The listing builds one solid part. Answer for the finished solid, in the listing's coordinates (mm). A direction names the side the tool comes from. Round coordinates to 2 decimals unless told otherwise and drop trailing zeros. Loops run counter-clockwise (first coordinate to the right, second up) from the corner with the lowest first, then second, coordinate; pieces in that order, holes last. Notation, with made-up numbers: (-12, 4.5) - (26, 4.5) arc R36 cw to (26, 43.5) - close; hole circle Ø9 at (-30, 62). An arc over 180 degrees is marked (long way). One line per item, written item: value.
```python
from build123d import *

# Parameters (mm, degrees)
PAD001_DEPTH  = 50
PAD002_DEPTH  = 50
SKETCH005_W   = 14
SKETCH005_H   = 13
PAD004_DEPTH  = 20
SKETCH006_W   = 14
SKETCH006_H   = 13
PAD005_DEPTH  = 20
SKETCH007_W   = 14
SKETCH007_H   = 13
PAD006_DEPTH  = 20
SKETCH008_W   = 14
SKETCH008_H   = 13
PAD007_DEPTH  = 20
SKETCH003_W   = 32
SKETCH003_H   = 3
PAD003_DEPTH  = 50
SKETCH004_R   = 2.75
HOLE_DEPTH    = 3.001
SKETCH009_W   = 16
SKETCH009_H   = 29
PAD008_DEPTH  = 30
SKETCH010_R   = 6.6
HOLE001_DEPTH = 29.001
SKETCH011_W   = 16
SKETCH011_H   = 29
PAD009_DEPTH  = 24
SKETCH012_R   = 6.6
HOLE002_DEPTH = 29.001001
SKETCH_W      = 32
SKETCH_H      = 42
PAD_DEPTH     = 50
SKETCH014_R   = 6.6
HOLE004_DEPTH = 32.001
FILLET_R      = 8
FILLET001_R   = 8


with BuildPart() as body001:
    # Sketch001 (on Face1 of CopyPad) → Pad001 (new body)
    with BuildSketch(Plane.YZ.offset(50)):
        Polygon((19, 44), (32, 44), (32, 2), (27, 2), (19, 12.011942), align=None)
    extrude(amount=-PAD001_DEPTH)


with BuildPart() as body002:
    # Sketch002 (on Face1 of CopyPad001) → Pad002 (new body)
    with BuildSketch(Plane.YZ.offset(50)):
        Polygon((13, 44), (13, 12), (5, 2), (0, 2), (0, 44), align=None)
    extrude(amount=-PAD002_DEPTH)


with BuildPart() as body004:
    # Sketch005 (on Face1 of CopyHole) → Pad004 (new body)
    with BuildSketch(Plane.XY.offset(2)):
        with Locations((7, 6.5)):
            Rectangle(SKETCH005_W, SKETCH005_H)
    extrude(amount=PAD004_DEPTH)


with BuildPart() as body005:
    # Sketch006 (on Face1 of CopyHole001) → Pad005 (new body)
    with BuildSketch(Plane.XY.offset(2)):
        with Locations((7, 25.5)):
            Rectangle(SKETCH006_W, SKETCH006_H)
    extrude(amount=PAD005_DEPTH)


with BuildPart() as body006:
    # Sketch007 (on Face1 of CopyHole002) → Pad006 (new body)
    with BuildSketch(Plane.XY.offset(2)):
        with Locations((43, 6.5)):
            Rectangle(SKETCH007_W, SKETCH007_H)
    extrude(amount=PAD006_DEPTH)


with BuildPart() as body007:
    # Sketch008 (on Face1 of CopyHole003) → Pad007 (new body)
    with BuildSketch(Plane.XY.offset(2)):
        with Locations((43, 25.5)):
            Rectangle(SKETCH008_W, SKETCH008_H)
    extrude(amount=PAD007_DEPTH)


with BuildPart() as body003:
    # Sketch003 (on Face1 of CopyPad002) → Pad003 (new body)
    with BuildSketch(Plane(origin=(0, 0, 0), x_dir=(0, -1, 0), z_dir=(-1, 0, 0))):
        with Locations((-16, 0.5)):
            Rectangle(SKETCH003_W, SKETCH003_H)
    extrude(amount=-PAD003_DEPTH)

    # Sketch004 (on Face1 of Pad003) → Hole (cut, through all)
    with BuildSketch(Plane.XY.offset(2)):
        with Locations((5, 27)):
            Circle(SKETCH004_R)
        with Locations((5, 5)):
            Circle(SKETCH004_R)
        with Locations((45, 5)):
            Circle(SKETCH004_R)
        with Locations((45, 27.276354)):
            Circle(SKETCH004_R)
    extrude(amount=-HOLE_DEPTH, mode=Mode.SUBTRACT)


with BuildPart() as body008:
    # Sketch009 (on Face1 of CopyPad003) → Pad008 (new body)
    with BuildSketch(Plane(origin=(0, 0, 44), x_dir=(0, -1, 0), z_dir=(0, 0, 1))):
        with Locations((-16, 24.5)):
            Rectangle(SKETCH009_W, SKETCH009_H)
    extrude(amount=PAD008_DEPTH)

    # Sketch010 (on Face1 of Pad008) → Hole001 (cut, through all)
    with BuildSketch(Plane(origin=(10, 0, 0), x_dir=(0, 1, 0), z_dir=(-1, 0, 0))):
        with Locations((16, -59)):
            Circle(SKETCH010_R)
    extrude(amount=-HOLE001_DEPTH, mode=Mode.SUBTRACT)


with BuildPart() as body009:
    # Sketch011 (on Face1 of CopyHole001001) → Pad009 (new body)
    with BuildSketch(Plane.XY.offset(74)):
        with Locations((25, 16)):
            Rectangle(SKETCH011_W, SKETCH011_H)
    extrude(amount=PAD009_DEPTH)

    # Sketch012 (on Face1 of Pad009) → Hole002 (cut, through all)
    with BuildSketch(Plane(origin=(-1e-06, 30.5, 30.000001), x_dir=(-1, 0, 0), z_dir=(0, 1, 0))):
        with Locations((-25, 59)):
            Circle(SKETCH012_R)
    extrude(amount=-HOLE002_DEPTH, mode=Mode.SUBTRACT)


with BuildPart() as body:
    # Sketch → Pad (new body)
    with BuildSketch(Plane.YZ):
        with Locations((16, 23)):
            Rectangle(SKETCH_W, SKETCH_H)
    extrude(amount=PAD_DEPTH)

    # Sketch014 (on Face2 of Pad) → Hole004 (cut, through all)
    with BuildSketch(Plane.ZX.offset(32)):
        with Locations((28.082674, 37)):
            Circle(SKETCH014_R)
        with Locations((28, 13)):
            Circle(SKETCH014_R)
    extrude(amount=-HOLE004_DEPTH, mode=Mode.SUBTRACT)

    # Boolean: cut Body001
    add(body001.part, mode=Mode.SUBTRACT)

    # Boolean001: cut Body002
    add(body002.part, mode=Mode.SUBTRACT)

    # Boolean002: cut Body004
    add(body004.part, mode=Mode.SUBTRACT)

    # Boolean003: cut Body005
    add(body005.part, mode=Mode.SUBTRACT)

    # Boolean004: cut Body006
    add(body006.part, mode=Mode.SUBTRACT)

    # Boolean005: cut Body007
    add(body007.part, mode=Mode.SUBTRACT)

    # Boolean006: union Body003
    add(body003.part)

    # Boolean007: union Body008, Body009
    add(body008.part)
    add(body009.part)

    # Fillet
    fillet_edges = [body.edges().sort_by_distance(p)[0] for p in [
        (50, 16, 44),
    ]]
    fillet(fillet_edges, radius=FILLET_R)

    # Fillet001
    fillet001_edges = [body.edges().sort_by_distance(p)[0] for p in [
        (0, 16, 44),
    ]]
    fillet(fillet001_edges, radius=FILLET001_R)


solid = body.part
```
1) A cutting plane is placed at A-A on x = 13. Give the vertices of the cut face in (y, z), and give its area (3 significant figures).
Final values:
outline: (0, -1) - (32, -1) - (32, 2) - (19, 2) - (19, 21.4) - (13, 21.4) - (13, 2) - (0, 2) - close; (8, 44) - (13, 44) - (13, 34.6) - (19, 34.6) - (19, 44) - (24, 44) - (24, 74) - (8, 74) - close; hole circle Ø13.2 at (16, 59)
area: 612 mm2
2) Consider L1, parallel to Z at x = 37, y = 16.25; L2, parallel to Y at x = 45, z = 0.85; L3, parallel to Z at x = 25.5, y = 27. Determine where each line is inside the solid, lowest interval first.
Final values:
L1: -1 to 21.48, 34.68 to 52.4, 65.6 to 74
L2: 0 to 2.25, 7.75 to 24.53, 30.03 to 32
L3: -1 to 2, 74 to 82.42, 95.58 to 98
3) For faces 4 (the flat face through (24, 24, 59)), 5 (the flat face through (36, 22, 6)), 6 (the flat face through (25, 5, 74)), determine the directions among +Z, -Z, +X, -X, +Y, -Y from which every point of the face is accessible in a straight line to the end or side of a thin tool.
Final values:
face 4: +X, -X, +Y
face 5: +X, +Y
face 6: +X, -X, -Y
4) For a pull along Z with two mould halves and no side action, classify faces 1 (the flat face through (25, 16, 98)), 2 (the flat face through (25, 28, 2)), 3 (the flat face through (50, 16, 13)) as released by +Z, released by -Z, zero draft, split by the parting line, or undercut.
Final values:
face 1: released by +Z
face 2: undercut
face 3: zero draft
5) A cutting plane is placed at B-B on z = 59. Give the vertices of the cut face in (x, y).
Final values:
outline: (10, 8) - (39, 8) - (39, 9.4) - (10, 9.4) - close; (10, 22.6) - (39, 22.6) - (39, 24) - (10, 24) - close
6) A cutting plane is placed at C-C on y = 21. Give the vertices of the cut face in (x, z), and give its area (3 significant figures).
Final values:
outline: (0, -1) - (50, -1) - (50, 2) - (36, 2) - (36, 9.51) - (14, 9.51) - (14, 2) - (0, 2) - close; (10, 44) - (39, 44) - (39, 54.69) - (10, 54.69) - close; (10, 63.31) - (39, 63.31) - (39, 74) - (33, 74) - (33, 98) - (17, 98) - (17, 74) - (10, 74) - close; hole circle Ø13.2 at (25, 89)
area: 1,180 mm2
7) Each of these flat-tipped pins is pushed along its axis until it touches: pin 1 Ø5 at (x, z) = (24, 73) entering from +Y; pin 2 Ø10.5 at (x, z) = (37, 28.08) entering from -Y (1 decimal); pin 3 Ø6.5 at (y, z) = (8.5, 5.5) entering from -X; pin 4 Ø6 at (x, z) = (26.5, 40.5) entering from -Y. Where does it stop, or does it pass through?
Final values:
pin 1: y = 30.5
pin 2: through
pin 3: x = 14
pin 4: y = 13
8) A cutting plane is placed at D-D on x = 40.5. Give the vertices of the cut face in (y, z), and give its area (3 significant figures).
Final values:
outline: (0, -1) - (32, -1) - (32, 2) - (19, 2) - (19, 22.49) - (13, 22.49) - (13, 2) - (0, 2) - close; (13, 33.68) - (19, 33.68) - (19, 44) - (13, 44) - close
area: 281 mm2
